Work out the finished part from the listing and answer in its coordinate system (mm). A direction names the side the tool comes from. Give positions to 0.01 mm unless a question says otherwise; leave off trailing zeros. Order: outer loops, then holes, each group sorted by start corner. A loop starts at its lowest first (then second) coordinate and runs counter-clockwise, first axis right, second up. Notation, with made-up numbers: (22, 78) -> (49, 78) arc R25 ccw to (49, 101) -> close; hole circle Ø7 at (-28.75, -34). An arc over 180 degrees is marked (long way). Answer as CSV lines item,"result". Start each with the question number.
1. A cutting plane is placed at A-A (y = 0). Give the vertices of the cut face in (x, z), then the cut area to 3 significant figures.
2. For a pull along X with two mould halves and no side action, classify faces 1 (the flat face through (32, -99, 58)), 2 (the cylindrical face through (105.874, 33.341, 27.608)), 3 (the cylindrical face through (-22.22, -100.063, 28.594)) as released by +X, released by -X, zero draft, split by the parting line, or undercut.
3. For faces 4 (the cylindrical face through (144.524, 45.513, 56.986)), 5 (the flat face through (-79, 79, 56)), determine the directions among +Z, -Z, +X, -X, +Y, -Y from which every point of the face is accessible in a straight line to the end or side of a thin tool.
4. A cutting plane is placed at D-D (y = 124). Give the vertices of the cut face in (x, z).
5. Find the intervals of material crossed by L1, parallel to X at y = 94.5, z = 47.5; L2, parallel to Y at x = 0, z = 32.5; L3, parallel to Z at x = -110, y = 18, in increasing order.
6. Flat-ended cylindrical pins translate along their axes: pin 1 (1.5 mm diameter, centred on x = 14.5, z = 51.5, fed in from -Y); pin 2 (1.5 mm diameter, centred on x = -46.5, z = 51.5, fed in from +Y); pin 3 (1.5 mm diameter, centred on y = -85.5, z = 13, fed in from -X). Find the tip coordinate at first contact, or state that the pin passes through.
7. A cutting plane is placed at C-C (z = 12.5). Give the vertices of the cut face in (x, y).
from build123d import *

# Parameters (mm, degrees)
SKETCH1_R           = 111
SKETCH1_R_2         = 102.5
BOSS_EXTRUDE1_DEPTH = 56
SKETCH2_R           = 2.544731427
CUT_EXTRUDE1_DEPTH  = 15
CIRPATTERN1_COUNT   = 8
SKETCH3_R           = 151.521158387
SKETCH3_R_2         = 102.5
BOSS_EXTRUDE2_DEPTH = 2


with BuildPart() as part:
    # Sketch1 → Boss-Extrude1 (new body)
    with BuildSketch(Plane.XY):
        Circle(SKETCH1_R)
        Circle(SKETCH1_R_2, mode=Mode.SUBTRACT)
    extrude(amount=BOSS_EXTRUDE1_DEPTH)

    # Sketch2 → Cut-Extrude1 (cut)
    with BuildSketch(Plane.XY.offset(56)):
        with Locations((29.439514058, 102.263864137)):
            Circle(SKETCH2_R)
    cut_extrude1 = extrude(amount=-CUT_EXTRUDE1_DEPTH, mode=Mode.SUBTRACT)

    # CirPattern1: Cut-Extrude1 ×8 about axis
    cirpattern1_axis = Axis((0, 0, 0), (0, 0, 1))
    for i in range(1, CIRPATTERN1_COUNT):
        add(cut_extrude1.rotate(cirpattern1_axis, i * 360 / CIRPATTERN1_COUNT), mode=Mode.SUBTRACT)

    # Sketch3 → Boss-Extrude2 (add)
    with BuildSketch(Plane.XY.offset(56)):
        Circle(SKETCH3_R)
        Circle(SKETCH3_R_2, mode=Mode.SUBTRACT)
    extrude(amount=BOSS_EXTRUDE2_DEPTH)


solid = part.part
Answer sheet:
1,outline,"(-151.52, 56) -> (-111, 56) -> (-111, 0) -> (-102.5, 0) -> (-102.5, 58) -> (-151.52, 58) -> close; (102.5, 0) -> (111, 0) -> (111, 56) -> (151.52, 56) -> (151.52, 58) -> (102.5, 58) -> close"
1,area,"1,150 mm^2"
2,face 1,"zero draft"
2,face 2,"split by the parting line"
2,face 3,"undercut"
3,face 4,"+Z, -Z"
3,face 5,"-Z"
4,outline,"(-87.08, 56) -> (87.08, 56) -> (87.08, 58) -> (-87.08, 58) -> close"
5,L1,"x = -58.23 to -53.64, -49.35 to -39.7, 39.7 to 58.23"
5,L2,"y = -111 to -102.5, 102.5 to 111"
5,L3,"z = 56 to 58"
6,pin 1,"stops at y = -110.15"
6,pin 2,"stops at y = 101.13"
6,pin 3,"stops at x = -71.68"
7,outline,"circle Ø222 at (0, 0); hole circle Ø205 at (0, 0)"
